from build123d import *

# Parameters (mm, degrees)
BOSS_EXTRUDE1_DEPTH = 30
FILLET1_R           = 10
SKETCH2_R           = 7.5
CUT_EXTRUDE1_DEPTH  = 138.840487521
SKETCH3_R           = 12.5
SKETCH3_R_2         = 5
BOSS_EXTRUDE2_DEPTH = 25


with BuildPart() as part:
    # Sketch1 → Boss-Extrude1 (new body)
    with BuildSketch(Plane.XY):
        Polygon((0, 0), (0, 100), (90, 100), (90, 0), (70, 0), (70, 80), (20, 80), (20, 0), align=None)
    extrude(amount=BOSS_EXTRUDE1_DEPTH)

    # Fillet1
    fillet1_edges = [part.edges().sort_by_distance(p)[0] for p in [
        (0, 100, 15),
        (90, 100, 15),
        (70, 80, 15),
        (20, 80, 15),
    ]]
    fillet(fillet1_edges, radius=FILLET1_R)

    # Sketch2 → Cut-Extrude1 (cut, through all)
    with BuildSketch(Plane(origin=(90, 0, 0), x_dir=(0, 0, -1), z_dir=(1, 0, 0))):
        with Locations(Location((-15, 25.249892163, 0), (0, 0, 90))):
            Circle(SKETCH2_R)
    extrude(amount=-CUT_EXTRUDE1_DEPTH, mode=Mode.SUBTRACT)

    # Sketch3 → Boss-Extrude2 (add)
    with BuildSketch(Plane(origin=(0, 100, 0), x_dir=(1, 0, 0), z_dir=(0, 1, 0))):
        with Locations(Location((45, -15, 0), (0, 0, 90))):
            Circle(SKETCH3_R)
        with Locations(Location((45, -15, 0), (0, 0, 270))):
            Circle(SKETCH3_R_2, mode=Mode.SUBTRACT)
    extrude(amount=BOSS_EXTRUDE2_DEPTH)


solid = part.part
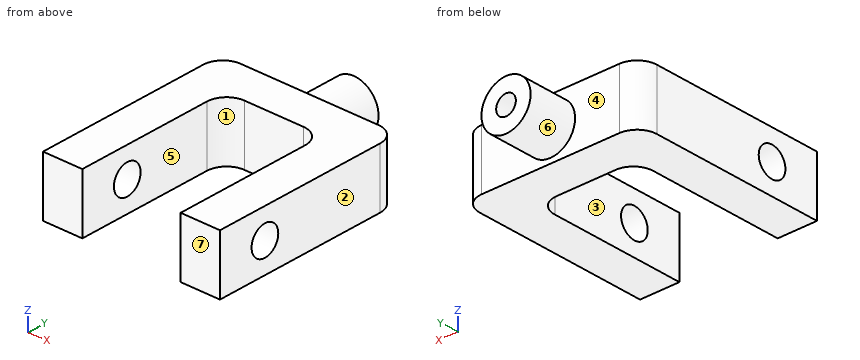
Geometry: final body of the model. Coordinates: model frame, mm. Face numbers are marked on the shaded views. A direction names the side the tool comes from. Give positions to 0.01 mm unless a question says otherwise; leave off trailing zeros. Write each loop counter-clockwise with the first axis right and the second up, starting at its lowest first coordinate (ties: lowest second). Pieces come first, ordered by that corner, then holes. Notation, with made-up numbers: (57, 3.5) - (108, 3.5) arc R27 cw to (108, 20.5) - close; hole circle Ø9 at (-15.75, -22.5). An arc over 180 degrees is marked (long way). Return JSON: item names as keys, results as strings. Group by question number.
1) Set-up query: the marked faces 5, 6 and 7. Return all of +Z, -Z, +X, -X, +Y, -Y with unobstructed straight access to the full face (end or side cutting, diameter ignored); none if empty.
2) Section D-D on z = 4. Return the cut outline in (x, y), plus the area to 3 significant figures.
3) First-contact query: P1, Ø1.5, axis at x = 25.5, z = 13, coming from the +Y side. Flat tip, straight axial feed; report the tip coordinate or a pass-through.
4) Line query: line 1 (X direction, y = 113, z = 15); line 2 (X direction, y = 60, z = 9); line 3 (Y direction, x = 36.5, z = 18). Output: solid intervals per line, ascending.
5) Section C-C on x = 45. Return the cut outline in (y, z), plus the area to 3 significant figures.
6) Mould query, pull axis X, two halves, no side actions, for the marked faces 1, 2, 3 and 4. Classes: released by +X, released by -X, zero draft, split by the parting line, or undercut.
7) Section B-B on y = 13.5. Return the cut outline in (x, z), plus the area to 3 significant figures.
8) Section A-A on z = 15. Return the cut outline in (x, y), plus the area to 4 significant figures.
Filled in:
{
 "1": {"face 5": "+Z, -Z, -Y", "face 6": "+Y", "face 7": "+Z, -Z, +X, -X, -Y"},
 "2": {"outline": "(0, 0) - (20, 0) - (20, 70) arc R10 cw to (30, 80) - (60, 80) arc R10 cw to (70, 70) - (70, 0) - (90, 0) - (90, 90) arc R10 ccw to (80, 100) - (50.94, 100) - (50.94, 125) - (39.06, 125) - (39.06, 100) - (10, 100) arc R10 ccw to (0, 90) - close", "area": "5,300 mm^2"},
 "3": {"P1": "stops at y = 100"},
 "4": {"line 1": "x = 32.5 to 40, 50 to 57.5", "line 2": "x = 0 to 20, 70 to 90", "line 3": "y = 80 to 125"},
 "5": {"outline": "(80, 0) - (100, 0) - (100, 2.5) - (125, 2.5) - (125, 10) - (100, 10) - (100, 20) - (125, 20) - (125, 27.5) - (100, 27.5) - (100, 30) - (80, 30) - close", "area": "975 mm^2"},
 "6": {"face 1": "undercut", "face 2": "released by +X", "face 3": "undercut", "face 4": "zero draft"},
 "7": {"outline": "(0, 0) - (20, 0) - (20, 30) - (0, 30) - close; (70, 0) - (90, 0) - (90, 30) - (70, 30) - close", "area": "1,200 mm^2"},
 "8": {"outline": "(0, 0) - (20, 0) - (20, 17.75) - (0, 17.75) - close; (0, 32.75) - (20, 32.75) - (20, 70) arc R10 cw to (30, 80) - (60, 80) arc R10 cw to (70, 70) - (70, 32.75) - (90, 32.75) - (90, 90) arc R10 ccw to (80, 100) - (57.5, 100) - (57.5, 125) - (50, 125) - (50, 100) - (40, 100) - (40, 125) - (32.5, 125) - (32.5, 100) - (10, 100) arc R10 ccw to (0, 90) - close; (70, 0) - (90, 0) - (90, 17.75) - (70, 17.75) - close", "area": "4,775 mm^2"}
}
